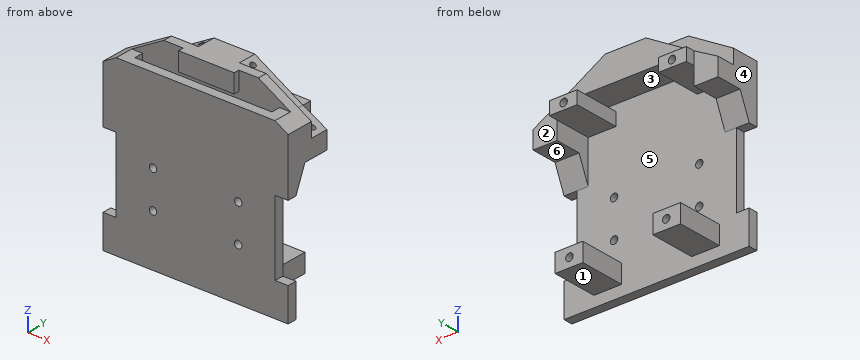
```python
from build123d import *

# Parameters (mm, degrees)
SKETCH1_R                = 2
BOSS_EXTRUDE1_DEPTH      = 5
SKETCH3_W                = 15
SKETCH3_H                = 7
SKETCH3_H_2              = 10
BOSS_EXTRUDE3_DEPTH      = 25
SKETCH4_R                = 2
CUT_EXTRUDE1_DEPTH       = 6
SKETCH8_W                = 45
SKETCH8_H                = 10
BOSS_EXTRUDE7_DEPTH      = 13
SKETCH17_W               = 100
SKETCH17_H               = 15
BOSS_EXTRUDE11_DEPTH     = 5
BOSS_EXTRUDE12_DEPTH     = 10
SKETCH19_W               = 13
SKETCH19_H               = 5
CUT_EXTRUDE7_DEPTH       = 10
CUT_EXTRUDE8_DEPTH       = 20
CUT_EXTRUDE9_DEPTH       = 120
BOSS_EXTRUDE13_DEPTH     = 20
CUT_EXTRUDE10_DEPTH      = 10
CUT_EXTRUDE10_DEPTH_BACK = 10
SKETCH22_R               = 1.5
CUT_EXTRUDE11_DEPTH      = 10
CUT_EXTRUDE11_DEPTH_BACK = 10
SKETCH24_R               = 1.5
SKETCH25_W               = 30
SKETCH25_H               = 10
BOSS_EXTRUDE14_DEPTH     = 3


with BuildPart() as part:
    # Sketch1 → Boss-Extrude1 (new body)
    with BuildSketch(Plane(origin=(0, 0, 0), x_dir=(1, 0, 0), z_dir=(0, 1, 0))):
        Polygon((-50, 40), (50, 40), (50, 22), (43, 22), (43, -18), (50, -18), (50, -53), (35, -53), (-35, -53), (-50, -53), (-50, -18), (-43, -18), (-43, 22), (-50, 22), align=None)
        with Locations(Location((-23, 12, 0), (0, 0, 270))):
            Circle(SKETCH1_R, mode=Mode.SUBTRACT)
        with Locations(Location((-23, -8, 0), (0, 0, 270))):
            Circle(SKETCH1_R, mode=Mode.SUBTRACT)
        with Locations(Location((23, -8, 0), (0, 0, 90))):
            Circle(SKETCH1_R, mode=Mode.SUBTRACT)
        with Locations(Location((23, 12, 0), (0, 0, 90))):
            Circle(SKETCH1_R, mode=Mode.SUBTRACT)
    extrude(amount=BOSS_EXTRUDE1_DEPTH)

    # Sketch3 → Boss-Extrude3 (add)
    with BuildSketch(Plane(origin=(0, 5, 0), x_dir=(1, 0, 0), z_dir=(0, 1, 0))):
        with Locations((-29.5, -44.5)):
            Rectangle(SKETCH3_W, SKETCH3_H)
        with Locations((-26.401946621, 29.165492724)):
            Rectangle(SKETCH3_W, SKETCH3_H_2)
        with Locations((29.5, -44.5)):
            Rectangle(SKETCH3_W, SKETCH3_H)
        with Locations((26.401946621, 29.165492724)):
            Rectangle(SKETCH3_W, SKETCH3_H_2)
    extrude(amount=BOSS_EXTRUDE3_DEPTH)

    # Sketch4 → Cut-Extrude1 (cut)
    with BuildSketch(Plane(origin=(0, 30, 0), x_dir=(1, 0, 0), z_dir=(0, 1, 0))):
        with Locations(Location((-29.25, -44.5, 0), (0, 0, 270))):
            Circle(SKETCH4_R)
        with Locations(Location((29.25, -44.5, 0), (0, 0, 270))):
            Circle(SKETCH4_R)
        with Locations(Location((-26.151946621, 29.165492724, 0), (0, 0, 270))):
            Circle(SKETCH4_R)
        with Locations(Location((26.151946621, 29.165492724, 0), (0, 0, 270))):
            Circle(SKETCH4_R)
    extrude(amount=-CUT_EXTRUDE1_DEPTH, mode=Mode.SUBTRACT)

    # Sketch8 → Boss-Extrude7 (add)
    with BuildSketch(Plane.ZY.offset(37)):
        with Locations((40.5, 10)):
            Rectangle(SKETCH8_W, SKETCH8_H)
    extrude(amount=BOSS_EXTRUDE7_DEPTH)

    # Mirror2: part across plane


with BuildPart() as part_1:
    add(part.part)
    add(part.part.mirror(Plane(origin=(0, 0, 0), x_dir=(0, 0, 1), z_dir=(1, 0, 0))))

    # Sketch17 → Boss-Extrude11 (add)
    with BuildSketch(Plane(origin=(0, 15, 0), x_dir=(1, 0, 0), z_dir=(0, 1, 0))):
        with Locations((0, -55.5)):
            Rectangle(SKETCH17_W, SKETCH17_H)
    extrude(amount=-BOSS_EXTRUDE11_DEPTH)

    # Sketch18 → Boss-Extrude12 (add)
    with BuildSketch(Plane(origin=(0, 15, 0), x_dir=(1, 0, 0), z_dir=(0, 1, 0))):
        Polygon((-37, -48), (-11.02885683, -63), (11.02885683, -63), (37, -48), align=None)
    extrude(amount=BOSS_EXTRUDE12_DEPTH)

    # Sketch19 → Cut-Extrude7 (cut)
    with BuildSketch(Plane.XY.offset(63)):
        with Locations((-43.5, 7.5)):
            Rectangle(SKETCH19_W, SKETCH19_H)
        with Locations((43.5, 7.5)):
            Rectangle(SKETCH19_W, SKETCH19_H)
    extrude(amount=-CUT_EXTRUDE7_DEPTH, mode=Mode.SUBTRACT)

    # Sketch20 → Cut-Extrude8 (cut)
    with BuildSketch(Plane(origin=(0, 15, 0), x_dir=(1, 0, 0), z_dir=(0, 1, 0))):
        Polygon((-25.568008611, -63), (-50, -48.888958818), (-50, -63), align=None)
        Polygon((50, -48.888958818), (50, -63), (25.568008611, -63), align=None)
    extrude(amount=-CUT_EXTRUDE8_DEPTH, mode=Mode.SUBTRACT)

    # Sketch21 → Cut-Extrude9 (cut)
    with BuildSketch(Plane(origin=(50, 0, 0), x_dir=(0, 0, -1), z_dir=(1, 0, 0))):
        Polygon((-41, 15), (-18, 5), (-18, 15), align=None)
    extrude(amount=-CUT_EXTRUDE9_DEPTH, mode=Mode.SUBTRACT)

    # Sketch23 → Boss-Extrude13 (add)
    with BuildSketch(Plane(origin=(0, 25, 0), x_dir=(1, 0, 0), z_dir=(0, 1, 0))):
        Polygon((-37, -48), (-50, -41), (-50, -31.394208948), (-37, -31.394208948), align=None)
        Polygon((50, -31.394208948), (37, -31.394208948), (37, -48), (50, -41), align=None)
    extrude(amount=-BOSS_EXTRUDE13_DEPTH)

    # Sketch22 → Cut-Extrude10 (cut, two sides: drawn at the far end of the back side and taken through both)
    with BuildSketch(Plane(origin=(-30.043596157, 0, 52.017769143), x_dir=(0.8659452125260777, 0, 0.5001388696183953), z_dir=(-0.5001388696183953, 0, 0.8659452125260777)).offset(-CUT_EXTRUDE10_DEPTH_BACK)):
        with Locations((-18.791636985, 20.670945853)):
            Circle(SKETCH22_R)
        with Locations(Location((18.208363015, 20.670945853, 0), (0, 0, 180))):
            Circle(SKETCH22_R)
    extrude(amount=CUT_EXTRUDE10_DEPTH + CUT_EXTRUDE10_DEPTH_BACK, mode=Mode.SUBTRACT)

    # Sketch24 → Cut-Extrude11 (cut, two sides: drawn at the far end of the back side and taken through both)
    with BuildSketch(Plane(origin=(30.043596157, 0, 52.017769143), x_dir=(0.8659452125260774, 0, -0.5001388696183958), z_dir=(0.5001388696183958, 0, 0.8659452125260774)).offset(-CUT_EXTRUDE11_DEPTH_BACK)):
        with Locations(Location((-18.208363015, 19.924140623, 0), (0, 0, 180))):
            Circle(SKETCH24_R)
        with Locations(Location((18.791636985, 19.924140623, 0), (0, 0, 180))):
            Circle(SKETCH24_R)
    extrude(amount=CUT_EXTRUDE11_DEPTH + CUT_EXTRUDE11_DEPTH_BACK, mode=Mode.SUBTRACT)

    # Sketch25 → Boss-Extrude14 (add)
    with BuildSketch(Plane.XZ.offset(-10)):
        with Locations((0, 58)):
            Rectangle(SKETCH25_W, SKETCH25_H)
    extrude(amount=BOSS_EXTRUDE14_DEPTH)


solid = part_1.part
```
Verification items for the finished model (mm, model axes). Face numbers are marked on the shaded views. A direction names the side the tool comes from. Round coordinates to 2 decimals unless told otherwise and drop trailing zeros. Order: outer loops, then holes, each group sorted by start corner. A loop starts at its lowest first (then second) coordinate and runs counter-clockwise, first axis right, second up. Notation, with made-up numbers: (32, 14) -> (68, 14) arc R21 cw to (68, 30) -> close; hole circle Ø7 at (18.5, 83). An arc over 180 degrees is marked (long way). Put each result on its own line as item: value. Start each with the question number.
(1) Tool access check on the marked faces 1, 2 and 3. Record the directions out of +Z, -Z, +X, -X, +Y, -Y that give a thin tool (end or side, any length) a straight path to the whole face; none if there is none.
(2) Section check A-A (z = -12). Enter the section's corners in (x, y), then the cut area to 3 significant figures.
(3) Depth check by flat-ended pin: pin 1 Ø3.5 at (x, z) = (-23, -12) entering from -Y; pin 2 Ø4 at (x, z) = (-36, 2.5) entering from +Y; pin 3 Ø10.5 at (x, z) = (43.5, 43) entering from +Y; pin 4 Ø16.5 at (x, y) = (24.5, 23.5) entering from +Z. Enter the tip coordinate at first touch or a pass-through.
(4) Draft check along Z on the marked faces 4, 5 and 6. Enter one of: +Z half, -Z half, draft (parallel to the pull), parting line (faces both ways), or undercut.
(5) Section check C-C (x = -4). Enter the section's corners in (y, z).
(6) Section check B-B (y = 13.5). Enter the section's corners in (x, z), then the cut area to 3 significant figures.
(7) Material ranges on line 1 along Z through (x, y) = (23, 1.7); line 2 along X through (y, z) = (28.2, 44.5); line 3 along Y through (x, z) = (26.5, 25), recorded low to high.
Completed:
1. face 1: -Z, +X, -X, +Y
1. face 2: +Z, -Z, +X, +Y
1. face 3: +Y
2. outline: (-43, 0) -> (-25, 0) -> (-25, 5) -> (-43, 5) -> close; (-21, 0) -> (21, 0) -> (21, 5) -> (-21, 5) -> close; (25, 0) -> (43, 0) -> (43, 5) -> (25, 5) -> close
2. area: 390 mm2
3. pin 1: passes through
3. pin 2: stops at y = 5
3. pin 3: stops at y = 25
3. pin 4: stops at z = 59.98
4. face 4: draft
4. face 5: undercut
4. face 6: -Z half
5. outline: (0, -40) -> (5, -40) -> (5, 53) -> (0, 53) -> close; (7, 53) -> (10, 53) -> (10, 48) -> (25, 48) -> (25, 63) -> (7, 63) -> close
6. outline: (-50, 31.39) -> (-37, 31.39) -> (-37, 41) -> (-22, 41) -> (-22, 48) -> (22, 48) -> (22, 41) -> (37, 41) -> (37, 31.39) -> (50, 31.39) -> (50, 48.89) -> (25.57, 63) -> (-25.57, 63) -> (-50, 48.89) -> close; (-33.9, -34.17) -> (-18.9, -34.17) -> (-18.9, -24.17) -> (-33.9, -24.17) -> close; (18.9, -34.17) -> (33.9, -34.17) -> (33.9, -24.17) -> (18.9, -24.17) -> close
6. area: 2,100 mm2
7. line 1: z = -40 to -14, -10 to 6, 10 to 53
7. line 2: x = -37 to -31.25, -27.25 to -22, 22 to 27.25, 31.25 to 37
7. line 3: y = 0 to 5
